Geometry: final body of the model. Coordinates: model frame, mm. Face numbers are marked on the shaded views. A direction names the side the tool comes from. Give positions to 0.01 mm unless a question says otherwise; leave off trailing zeros. Order: outer loops, then holes, each group sorted by start corner. A loop starts at its lowest first (then second) coordinate and runs counter-clockwise, first axis right, second up. Notation, with made-up numbers: (44, 34) - (92, 34) arc R20 cw to (92, 51) - close; hole circle Ø8 at (41, 33). An arc over 180 degrees is marked (long way). Put each result on its own line as item: value. Start each with the question number.
1. Section D-D on z = -3.5. Return the cut outline in (x, y), plus the area to 3 significant figures.
2. Section B-B on z = -35.5. Return the cut outline in (x, y), plus the area to 3 significant figures.
3. Ray query, line 1 along X through (y, z) = (9, -31); line 2 along Y through (x, z) = (75, -11); line 3 along Z through (x, y) = (25, 8). Return the intervals inside material, ascending. Write a range as from..to.
4. Section A-A on x = 25. Return the cut outline in (y, z), plus the area to 3 significant figures.
5. Mould query, pull axis Y, two halves, no side actions, for the marked faces 6, 7 and 8. Classes: pulls with the +Y half, pulls with the -Y half, needs draft (parallel to the pull), parting line crosses it, or undercut.
6. Set-up query: the marked faces 1, 2, 3, 4 and 5. Return all of +Z, -Z, +X, -X, +Y, -Y with unobstructed straight access to the full face (end or side cutting, diameter ignored); none if empty.
7. First-contact query: P1, Ø1.5, axis at x = 83, y = 109, coming from the -Z side; P2, Ø4, axis at x = 29, z = -42, coming from the +Y side; P3, Ø2, axis at y = 37.5, z = -35, coming from the -X side. Flat tips, straight axial feed; report the tip coordinate or a pass-through.
8. Section C-C on y = 51. Return the cut outline in (x, z), plus the area to 3 significant figures.
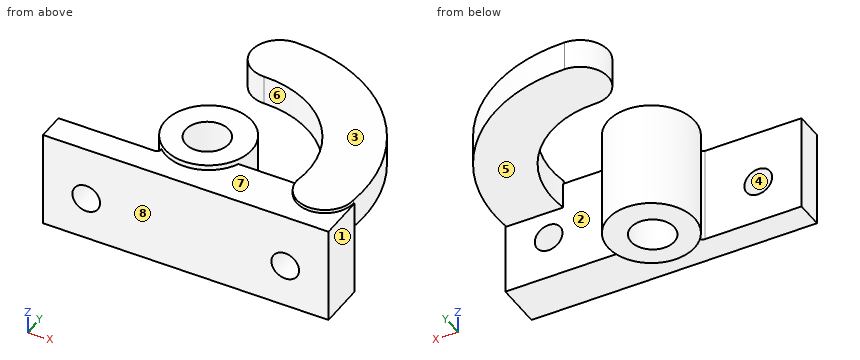
from build123d import *

# Parameters (mm, degrees)
SKETCH1_W                = 165
SKETCH1_H                = 56
BOSS_EXTRUDE1_DEPTH      = 16
SKETCH2_R                = 8
CUT_EXTRUDE1_DEPTH       = 16
SKETCH3_R                = 25
BOSS_EXTRUDE2_DEPTH      = 3
BOSS_EXTRUDE2_DEPTH_BACK = 59
FILLET1_R                = 2
SKETCH4_R                = 12.5
CUT_EXTRUDE2_DEPTH       = 63
SKETCH5_W                = 76.508877986
SKETCH5_H                = 56
SKETCH5_R                = 8
BOSS_EXTRUDE3_DEPTH      = 11
BOSS_EXTRUDE5_DEPTH      = 2
BOSS_EXTRUDE5_DEPTH_BACK = 15


with BuildPart() as part:
    # Sketch1 → Boss-Extrude1 (new body)
    with BuildSketch(Plane(origin=(0, 0, 0), x_dir=(1, 0, 0), z_dir=(0, 1, 0))):
        with Locations((82.5, 28)):
            Rectangle(SKETCH1_W, SKETCH1_H)
    extrude(amount=BOSS_EXTRUDE1_DEPTH)

    # Sketch2 → Cut-Extrude1 (cut)
    with BuildSketch(Plane(origin=(0, 16, 0), x_dir=(1, 0, 0), z_dir=(0, 1, 0))):
        with Locations((25, 31)):
            Circle(SKETCH2_R)
        with Locations((140, 31)):
            Circle(SKETCH2_R)
    extrude(amount=-CUT_EXTRUDE1_DEPTH, mode=Mode.SUBTRACT)

    # Sketch3 → Boss-Extrude2 (add, two sides)
    with BuildSketch(Plane.XY) as boss_extrude2_sk:
        with Locations((75, 37.047318756)):
            Circle(SKETCH3_R)
    extrude(amount=BOSS_EXTRUDE2_DEPTH)
    extrude(boss_extrude2_sk.sketch, amount=-BOSS_EXTRUDE2_DEPTH_BACK)

    # Fillet1
    fillet1_edges = [part.edges().sort_by_distance(p)[0] for p in [
        (61.508877986, 16, -28),
    ]]
    fillet(fillet1_edges, radius=FILLET1_R)

    # Sketch4 → Cut-Extrude2 (cut, through all)
    with BuildSketch(Plane.XY.offset(3)):
        with Locations((75, 35.713660164)):
            Circle(SKETCH4_R)
    extrude(amount=-CUT_EXTRUDE2_DEPTH, mode=Mode.SUBTRACT)

    # Sketch5 → Boss-Extrude3 (add)
    with BuildSketch(Plane(origin=(0, 16, 0), x_dir=(1, 0, 0), z_dir=(0, 1, 0))):
        with Locations((126.745561007, 28)):
            Rectangle(SKETCH5_W, SKETCH5_H)
        with Locations((140, 31)):
            Circle(SKETCH5_R, mode=Mode.SUBTRACT)
    extrude(amount=BOSS_EXTRUDE3_DEPTH)

    # Sketch8 → Boss-Extrude5 (add, two sides)
    with BuildSketch(Plane.XY) as boss_extrude5_sk:
        with BuildLine():
            ThreePointArc((75, 127.047318756), (142.097908641, 97.029571598), (164.437416028, 27))
            ThreePointArc((164.437416028, 27), (148, 10.562583972), (131.562583972, 27))
            ThreePointArc((131.562583972, 27), (119.031085874, 73.946343086), (75, 94.495334559))
            ThreePointArc((75, 94.495334559), (58.724007902, 110.771326658), (75, 127.047318756))
        make_face()
    extrude(amount=BOSS_EXTRUDE5_DEPTH)
    extrude(boss_extrude5_sk.sketch, amount=-BOSS_EXTRUDE5_DEPTH_BACK)


solid = part.part
Resolved:
1. outline: (0, 0) - (165, 0) - (165, 27) - (164.44, 27) arc R90 ccw to (75, 127.05) arc R16.28 ccw to (75, 94.5) arc R57.45 cw to (131.56, 27) - (97.89, 27) arc R25 ccw (long way) to (57.28, 19.41) arc R2 cw to (55.86, 16) - (0, 16) - close; hole circle Ø25 at (75, 35.71)
1. area: 9,340 mm^2
2. outline: (0, 0) - (18.39, 0) - (18.39, 16) - (0, 16) - close; (31.61, 0) - (133.39, 0) - (133.39, 27) - (97.89, 27) arc R25 ccw (long way) to (57.28, 19.41) arc R2 cw to (55.86, 16) - (31.61, 16) - close; (146.61, 0) - (165, 0) - (165, 27) - (146.61, 27) - close; hole circle Ø25 at (75, 35.71)
2. area: 4,260 mm^2
3. line 1: 0..17, 33..132, 148..165
3. line 2: 0..23.21, 48.21..62.05, 94.5..127.05
3. line 3: -56..-39, -23..0
4. outline: (0, -56) - (16, -56) - (16, -39) - (0, -39) - close; (0, -23) - (16, -23) - (16, 0) - (0, 0) - close
4. area: 640 mm^2
5. face 6: undercut
5. face 7: needs draft
5. face 8: pulls with the -Y half
6. face 1: +Z, -Z, +X, +Y, -Y
6. face 2: -Z
6. face 3: +Z, +X, +Y
6. face 4: +Y, -Y
6. face 5: -Z, +X, +Y
7. P1: z = -15
7. P2: y = 16
7. P3: x = 50
8. outline: (54.26, -59) - (95.74, -59) - (95.74, 3) - (54.26, 3) - close; (130.73, -15) - (163.91, -15) - (163.91, 2) - (130.73, 2) - close
8. area: 3,140 mm^2
